Geometry check sheet. Reference: the model listing, model coordinates, mm. Face numbers are marked on the shaded views. A direction names the side the tool comes from. Coordinates: 2 decimals unless noted, no trailing zeros. Loops run counter-clockwise (first coordinate to the right, second up) from the corner with the lowest first, then second, coordinate; pieces in that order, holes last. Notation, with made-up numbers: (51.25, -34.5) -> (78.25, -34.5) arc R24 cw to (78.25, -2.5) -> close; hole circle Ø3 at (82.25, 13.5). An arc over 180 degrees is marked (long way). Answer as a JSON object with one key per item and string values.
from build123d import *

# Parameters (mm, degrees)
F0_W      = 43
F0_H      = 60
F1_DEPTH  = 37
F2_W      = 33
F2_H      = 50
F3_DEPTH  = 35
F5_DEPTH  = 10
F7_DEPTH  = 10
F9_DEPTH  = 10
F12_DEPTH = 14
F14_DEPTH = 14
F16_DEPTH = 14
F18_DEPTH = 14
F19_R     = 5
F20_DEPTH = 6
F22_DEPTH = 33
F23_DEPTH = 33
F24_DEPTH = 33
F25_DEPTH = 33
F26_R     = 3.000008
F27_DEPTH = 15
F28_R     = 3.025892
F29_DEPTH = 15
F30_R     = 3
F31_DEPTH = 15
F32_R     = 3
F33_DEPTH = 15
F34_DEPTH = 35
F35_R     = 3
F36_DEPTH = 10
F37_R     = 3.000007
F38_DEPTH = 10
F39_R     = 3.004044
F40_DEPTH = 10
F41_R     = 3.03892
F42_DEPTH = 10


with BuildPart() as f1:
    # F0 (on Top) → F1 (new body)
    with BuildSketch(Plane.XY):
        Rectangle(F0_W, F0_H)
    extrude(amount=F1_DEPTH)

    # F2 (on face) → F3 (cut)
    with BuildSketch(Plane.XY.offset(37)):
        Rectangle(F2_W, F2_H)
    extrude(amount=-F3_DEPTH, mode=Mode.SUBTRACT)

    # F4 (on face) → F5 (cut)
    with BuildSketch(Plane.XY.offset(37)):
        Polygon((11.5, 30), (0, 30), (-11.5, 30), (-11.5, 25), (0, 25), (11.5, 25), align=None)
    extrude(amount=-F5_DEPTH, mode=Mode.SUBTRACT)

    # F6 (on face) → F7 (join)
    with BuildSketch(Plane.XY.offset(27)):
        Polygon((2.5, 25), (0, 30), (-2.5, 25), (0, 25), align=None)
    extrude(amount=F7_DEPTH)

    # F8 (on face) → F9 (cut)
    with BuildSketch(Plane.XY.offset(37)):
        Polygon((5, -25), (0, -25), (-5, -25), (-5, -30), (0, -30), (5, -30), align=None)
    extrude(amount=-F9_DEPTH, mode=Mode.SUBTRACT)

    # F11 (on face) → F12 (join)
    with BuildSketch(Plane.XY.offset(2)):
        Polygon((8, 19), (0, 19), (-8, 19), (-8, 0), (-8, -8), (0, -8), (8, -8), (8, 0), align=None)
    extrude(amount=F12_DEPTH)

    # F13 (on face) → F14 (cut)
    with BuildSketch(Plane.XY.offset(16)):
        Polygon((6.5, 17), (0, 17), (-6.5, 17), (-6.5, 0), (-6.5, -6), (0, -6), (6.5, -6), (6.5, 0), align=None)
    extrude(amount=-F14_DEPTH, mode=Mode.SUBTRACT)

    # F15 (on face) → F16 (cut)
    with BuildSketch(Plane.XY.offset(16)):
        Polygon((3, 19), (0, 19), (-3, 19), (-3, 17), (0, 17), (3, 17), align=None)
    extrude(amount=-F16_DEPTH, mode=Mode.SUBTRACT)

    # F17 (on face) → F18 (cut)
    with BuildSketch(Plane.XY.offset(16)):
        Polygon((3, -6), (0, -6), (-3, -6), (-3, -8), (0, -8), (3, -8), align=None)
    extrude(amount=-F18_DEPTH, mode=Mode.SUBTRACT)

    # F19 (on face) → F20 (cut)
    with BuildSketch(Plane.XZ.offset(30)):
        with Locations((0, 7.785951)):
            Circle(F19_R)
    extrude(amount=-F20_DEPTH, mode=Mode.SUBTRACT)

    # F21 (on face) → F22 (join)
    with BuildSketch(Plane.XY.offset(37)):
        Polygon((-16.5, -10.623924), (-16.5, -17.623924), (-9.5, -17.623924), align=None)
    extrude(amount=-F22_DEPTH)

    # F21 (on face) → F23 (join)
    with BuildSketch(Plane.XY.offset(37)):
        Polygon((16.5, -17.623924), (16.5, -10.623924), (9.5, -17.623924), align=None)
    extrude(amount=-F23_DEPTH)

    # F21 (on face) → F24 (join)
    with BuildSketch(Plane.XY.offset(37)):
        Polygon((-9.5, 17.623924), (-16.5, 17.623924), (-16.5, 10.623924), align=None)
    extrude(amount=-F24_DEPTH)

    # F21 (on face) → F25 (join)
    with BuildSketch(Plane.XY.offset(37)):
        Polygon((9.5, 17.623924), (16.5, 10.623924), (16.5, 17.623924), align=None)
    extrude(amount=-F25_DEPTH)

    # F26 (on face) → F27 (cut)
    with BuildSketch(Plane.XZ.offset(17.623924)):
        with Locations((-13.006919, 32.922085)):
            Circle(F26_R)
    extrude(amount=-F27_DEPTH, mode=Mode.SUBTRACT)

    # F28 (on face) → F29 (cut)
    with BuildSketch(Plane.XZ.offset(17.623924)):
        with Locations((13.051108, 32.73694)):
            Circle(F28_R)
    extrude(amount=-F29_DEPTH, mode=Mode.SUBTRACT)

    # F30 (on face) → F31 (cut)
    with BuildSketch(Plane(origin=(0, 17.623924, 0), x_dir=(-1, 0, 0), z_dir=(0, 1, 0))):
        with Locations((-12.977869, 32.83175)):
            Circle(F30_R)
    extrude(amount=-F31_DEPTH, mode=Mode.SUBTRACT)

    # F32 (on face) → F33 (cut)
    with BuildSketch(Plane(origin=(0, 17.623924, 0), x_dir=(-1, 0, 0), z_dir=(0, 1, 0))):
        with Locations((13.297083, 33.348583)):
            Circle(F32_R)
    extrude(amount=-F33_DEPTH, mode=Mode.SUBTRACT)

    # F21 (on face) → F34 (join)
    with BuildSketch(Plane.XY.offset(37)):
        Polygon((-16.5, -10.623924), (-16.5, -17.623924), (-9.5, -17.623924), align=None)
        Polygon((16.5, -17.623924), (16.5, -10.623924), (9.5, -17.623924), align=None)
        Polygon((-9.5, 17.623924), (-16.5, 17.623924), (-16.5, 10.623924), align=None)
        Polygon((9.5, 17.623924), (16.5, 10.623924), (16.5, 17.623924), align=None)
    extrude(amount=-F34_DEPTH)

    # F35 (on face) → F36 (cut)
    with BuildSketch(Plane.XZ.offset(17.623924)):
        with Locations((-13.037096, 33.683364)):
            Circle(F35_R)
    extrude(amount=-F36_DEPTH, mode=Mode.SUBTRACT)

    # F37 (on face) → F38 (cut)
    with BuildSketch(Plane.XZ.offset(17.623924)):
        with Locations((12.993197, 33.357316)):
            Circle(F37_R)
    extrude(amount=-F38_DEPTH, mode=Mode.SUBTRACT)

    # F39 (on face) → F40 (cut)
    with BuildSketch(Plane(origin=(0, 17.623924, 0), x_dir=(-1, 0, 0), z_dir=(0, 1, 0))):
        with Locations((-12.973316, 33.344424)):
            Circle(F39_R)
    extrude(amount=-F40_DEPTH, mode=Mode.SUBTRACT)

    # F41 (on face) → F42 (cut)
    with BuildSketch(Plane(origin=(0, 17.623924, 0), x_dir=(-1, 0, 0), z_dir=(0, 1, 0))):
        with Locations((13.015212, 33.45837)):
            Circle(F41_R)
    extrude(amount=-F42_DEPTH, mode=Mode.SUBTRACT)


solid = f1.part
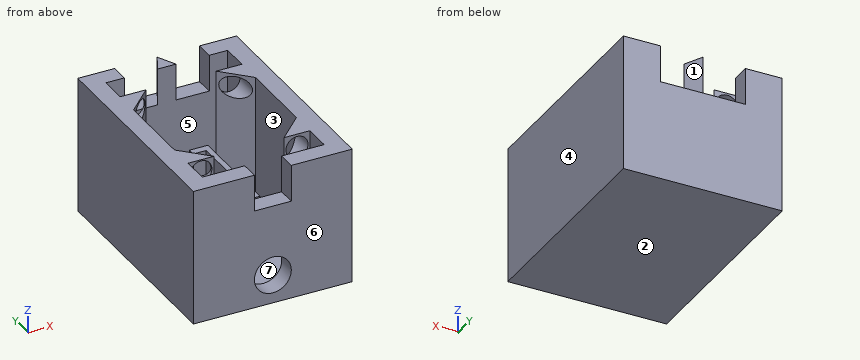
1. Tool access check on the marked faces 1, 2 and 3. Record the directions out of +Z, -Z, +X, -X, +Y, -Y that give a thin tool (end or side, any length) a straight path to the whole face; none if there is none.
Evaluation:
{"face 1": "+Z, +Y", "face 2": "-Z, +X, -X, +Y, -Y", "face 3": "+Z"}
2. Section check D-D, the plane y = 9.5. Record the boundary of the cut face in (x, z).
Evaluation:
{"outline": "(-21.5, 0) -> (21.5, 0) -> (21.5, 37) -> (16.5, 37) -> (16.5, 2) -> (8, 2) -> (8, 16) -> (6.5, 16) -> (6.5, 2) -> (-6.5, 2) -> (-6.5, 16) -> (-8, 16) -> (-8, 2) -> (-16.5, 2) -> (-16.5, 37) -> (-21.5, 37) -> close"}
3. Mould release check, pull along Y, two halves, no side actions. Record for the marked faces 4, 5, 6 and 7: released by +Y, released by -Y, zero draft, split by the parting line, or undercut.
Evaluation:
{"face 4": "zero draft", "face 5": "undercut", "face 6": "released by -Y", "face 7": "undercut"}
4. Section check A-A, the plane z = 26. Record the boundary of the cut face in (x, y).
Evaluation:
{"outline": "(-21.5, -30) -> (21.5, -30) -> (21.5, 30) -> (-21.5, 30) -> close; hole (-16.5, -25) -> (16.5, -25) -> (16.5, -17.62) -> (9.5, -17.62) -> (16.5, -10.62) -> (16.5, 10.62) -> (9.5, 17.62) -> (16.5, 17.62) -> (16.5, 25) -> (-16.5, 25) -> (-16.5, 17.62) -> (-9.5, 17.62) -> (-16.5, 10.62) -> (-16.5, -10.62) -> (-9.5, -17.62) -> (-16.5, -17.62) -> close"}
5. Thickness scan on probe 1 along X at (y, z) = (-1.5, 9.5); probe 2 along Y at (x, z) = (0, 21.5); probe 3 along X at (y, z) = (22, 24.5). Record the ranges inside material, lowest first. Write a range as from..to.
Evaluation:
{"probe 1": "x = -21.5..-16.5, -8..-6.5, 6.5..8, 16.5..21.5", "probe 2": "y = -30..-25, 25..30", "probe 3": "x = -21.5..-16.5, 16.5..21.5"}
6. Section check C-C, the plane z = 14. State how many separate pieces and enclosed holes the cut face has, then the cut area to 3 significant figures.
Evaluation:
{"separate pieces": "3", "enclosed holes": "1", "area": "1,140 mm^2"}
7. Depth check by flat-ended pin: P1, Ø4, axis at x = -5.5, y = 8.5, coming from the +Z side; P2, Ø6, axis at x = -3, y = 10, coming from the +Z side; P3, Ø5.5, axis at x = 8.5, y = 28, coming from the +Z side; P4, Ø11.5, axis at x = 0, z = 7.79, coming from the -Y side. Enter the tip coordinate at first touch or a pass-through.
Evaluation:
{"P1": "stops at z = 16", "P2": "stops at z = 2", "P3": "stops at z = 27", "P4": "stops at y = -30"}
8. Section check B-B, the plane y = 24. Record the boundary of the cut face in (x, z), then the cut area to 3 significant figures.
Evaluation:
{"outline": "(-21.5, 0) -> (21.5, 0) -> (21.5, 37) -> (16.5, 37) -> (16.5, 2) -> (-16.5, 2) -> (-16.5, 37) -> (-21.5, 37) -> close", "area": "436 mm^2"}
